Verification items for this drawing (mm, ordinates from the low corner). Coordinates: 2 decimals unless noted, no trailing zeros. Write each loop counter-clockwise with the first axis right and the second up, starting at its lowest first coordinate (ties: lowest second). Pieces come first, ordered by that corner, then holes.
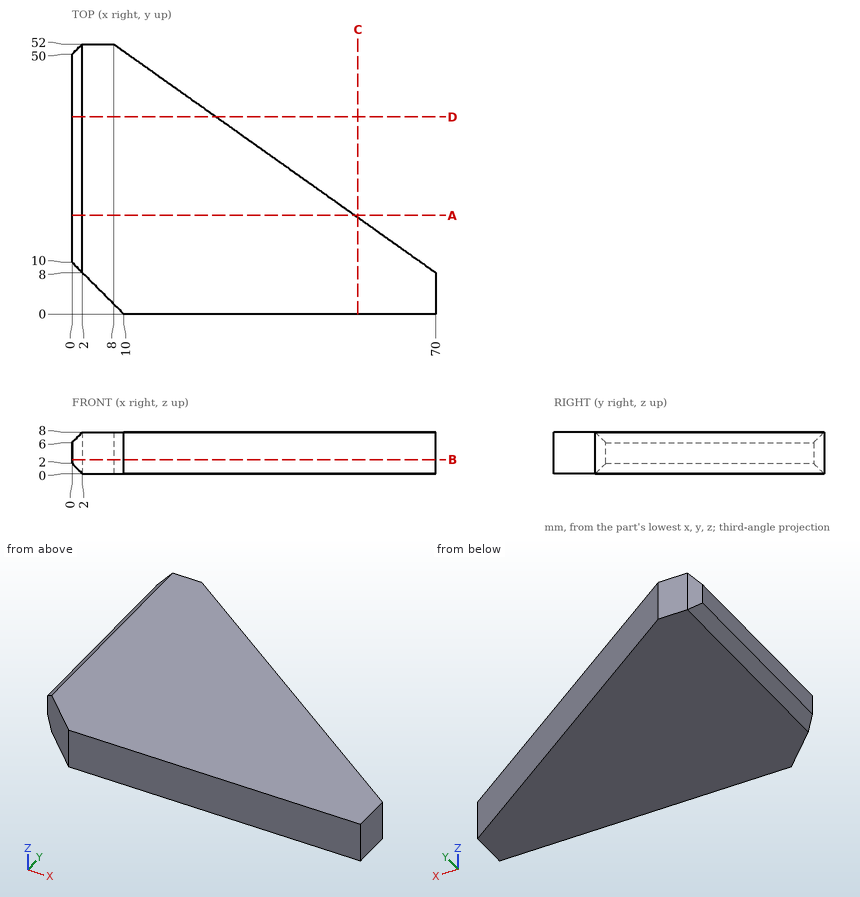
1. Sectioned sample at D-D, the plane y = 38. Record the boundary of the cut face in (x, z), and give its area (3 significant figures).
Computed values:
outline: (0, 2) - (2, 0) - (27.73, 0) - (27.73, 8) - (2, 8) - (0, 6) - close
area: 218 mm2
2. Sectioned sample at B-B, the plane z = 2.75. Record the boundary of the cut face in (x, y), and give its area (3 significant figures).
Computed values:
outline: (0, 10) - (10, 0) - (70, 0) - (70, 8) - (8, 52) - (2, 52) - (0, 50) - close
area: 2,220 mm2
3. Sectioned sample at C-C, the plane x = 55. Record the boundary of the cut face in (y, z).
Computed values:
outline: (0, 0) - (18.65, 0) - (18.65, 8) - (0, 8) - close
4. Sectioned sample at A-A, the plane y = 19. Record the boundary of the cut face in (x, z).
Computed values:
outline: (0, 2) - (2, 0) - (54.5, 0) - (54.5, 8) - (2, 8) - (0, 6) - close
5. Thickness scan on line 1 along Y through (x, z) = (14, 5); line 2 along Y through (x, z) = (46.5, 1.75); line 3 along X through (y, z) = (31.5, 6.25). Record the ranges inside material, lowest first.
Computed values:
line 1: y = 0 to 47.74
line 2: y = 0 to 24.68
line 3: x = 0.25 to 36.89
6. Gauge pin test, flat end, axial feed: pin 1 Ø1.5 at (x, y) = (32, 35) entering from +Z. Record the tip position at first contact, or that the pin passes through.
Computed values:
pin 1: stops at z = 8
